```python
from build123d import *

# Parameters (mm, degrees)
F0_W     = 130.376012
F0_H     = 71.088024
F1_DEPTH = 50.8
F2_T     = -5.08
F4_D     = 3.81


with BuildPart() as f1:
    # F0 (on Top) → F1 (new body)
    with BuildSketch(Plane.XY):
        Rectangle(F0_W, F0_H)
    extrude(amount=F1_DEPTH)

    # F2
    f2_openings = [f1.faces().sort_by_distance(p)[0] for p in [
        (0, 0, 50.8),
    ]]
    offset(amount=F2_T, openings=f2_openings)

    # F4 (through all)
    with Locations(Plane.YZ.offset(65.188006)):
        with Locations((-26.334226, 8.001857), (-20.002501, 8.001857), (-13.670773, 8.001857), (-6.475631, 8.001857), (0, 8.001857), (6.187825, 8.001857), (12.231745, 8.001857), (20.290304, 8.001857), (25.470806, 8.001857)):
            Hole(F4_D / 2)


solid = f1.part
```
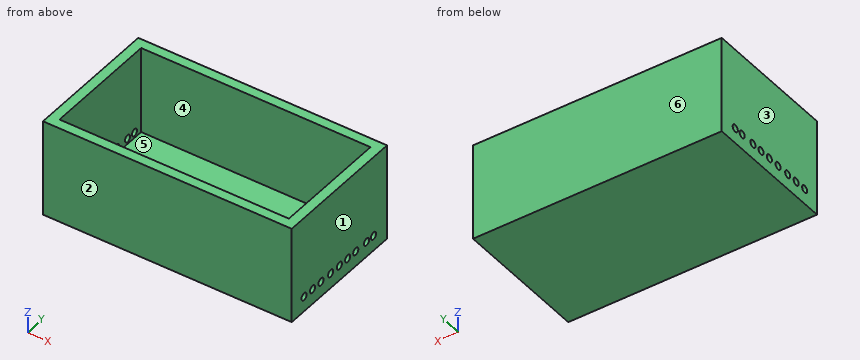
Source: CAD feature listing. Evaluate the final solid. Frame: model axes, mm. Face numbers are marked on the shaded views. A direction names the side the tool comes from. Give positions to 0.01 mm unless a question says otherwise; leave off trailing zeros. Loops run counter-clockwise (first coordinate to the right, second up) from the corner with the lowest first, then second, coordinate; pieces in that order, holes last. Notation, with made-up numbers: (-14.5, 86) - (-10.5, 86) arc R18 cw to (-10.5, 118) - close; hole circle Ø10 at (37.25, 74). An arc over 180 degrees is marked (long way). Use CSV: the item, a comma, the result in double quotes. Start each with the question number.
1. Section C-C (x = -51.5). Output: boundary loops of the cut face in (y, z).
2. Section A-A (z = 36.5). Output: boundary loops of the cut face in (x, y), then the cut area to 3 significant figures.
3. Pin query (flat end, axial travel): pin 1 (3 mm diameter, centred on y = 0, z = 8, fed in from +X); pin 2 (12 mm diameter, centred on x = -18, y = 5.5, fed in from -Z); pin 3 (10 mm diameter, centred on x = -22, y = 20.5, fed in from +Z). Return the tip coordinate at first contact, or that it passes through.
4. Draft query along X for the marked faces 1, 2, 3 and 4. Return one class per face: +X half, -X half, draft (parallel to the pull), parting line (faces both ways), or undercut.
5. Reachability of the marked faces 5 and 6 from +Z, -Z, +X, -X, +Y, -Y: full face, straight path, thin tool, end or side. Return the list, or none.
6. Section B-B (y = 0). Output: boundary loops of the cut face in (x, z), then the cut area to 3 significant figures.
7. Ray query, L1, parallel to X at y = 4.5, z = 28.5; L2, parallel to Y at x = 41, z = 22; L3, parallel to Z at x = 25.5, y = 28.5. Return the intervals inside material, ascending.
Response:
1,outline,"(-35.54, 0) - (35.54, 0) - (35.54, 50.8) - (30.46, 50.8) - (30.46, 5.08) - (-30.46, 5.08) - (-30.46, 50.8) - (-35.54, 50.8) - close"
2,outline,"(-65.19, -35.54) - (65.19, -35.54) - (65.19, 35.54) - (-65.19, 35.54) - close; hole (-60.11, -30.46) - (60.11, -30.46) - (60.11, 30.46) - (-60.11, 30.46) - close"
2,area,"1,940 mm²"
3,pin 1,"through"
3,pin 2,"z = 0"
3,pin 3,"z = 5.08"
4,face 1,"+X half"
4,face 2,"draft"
4,face 3,"-X half"
4,face 4,"undercut"
5,face 5,"+Z"
5,face 6,"+Z, -Z, +X, -X, +Y"
6,outline,"(-65.19, 0) - (65.19, 0) - (65.19, 6.1) - (60.11, 6.1) - (60.11, 5.08) - (-60.11, 5.08) - (-60.11, 6.1) - (-65.19, 6.1) - close; (-65.19, 9.91) - (-60.11, 9.91) - (-60.11, 50.8) - (-65.19, 50.8) - close; (60.11, 9.91) - (65.19, 9.91) - (65.19, 50.8) - (60.11, 50.8) - close"
6,area,"1,090 mm²"
7,L1,"-65.19 to -60.11, 60.11 to 65.19"
7,L2,"-35.54 to -30.46, 30.46 to 35.54"
7,L3,"0 to 5.08"
